Autodesk Inventor part; units mm, degrees
ref_plane "YZ Plane" through (0, 0, 0) normal (1, 0, 0) x (0, 1, 0)
ref_plane "XZ Plane" through (0, 0, 0) normal (0, 1, 0) x (-1, 0, 0)
ref_plane "XY Plane" through (0, 0, 0) normal (0, 0, 1) x (1, 0, 0)
sketch "Esquisse1" plane through (0, 0, 0) normal (0, 1, 0) x (-1, 0, 0)
  line L0 (-350, -500) -> (350, -500)
  line L1 (350, -500) -> (350, 500)
  line L2 (350, 500) -> (-350, 500)
  line L3 (-350, 500) -> (-350, -500)
  line L4 (-350, -500) -> (350, 500) construction
  line L5 (350, -500) -> (-350, 500) construction
  point P0 (0, 0)
  dimension "d0" = 1000
  dimension "d1" = 700
extrude "Extrusion1" add sketch "Esquisse1" along normal blind 18.55
sketch "Esquisse2" plane through (0, 18.55, 0) normal (0, 1, 0) x (1, 0, 0)
  line L0 (-350, 500) -> (-350, -500)
  line L1 (-350, -450) -> (-331.45, -450)
  line L2 (-331.45, -450) -> (-331.45, -350)
  line L3 (-331.45, -350) -> (-350, -350)
  line L4 (-350, -350) -> (-350, -450)
  line L5 (-350, -250) -> (-331.45, -250)
  line L6 (-331.45, -250) -> (-331.45, -150)
  line L7 (-331.45, -150) -> (-350, -150)
  line L8 (-350, -150) -> (-350, -250)
  line L9 (-350, -50) -> (-331.45, -50)
  line L10 (-331.45, -50) -> (-331.45, 50)
  line L11 (-331.45, 50) -> (-350, 50)
  line L12 (-350, 50) -> (-350, -50)
  line L13 (-350, 150) -> (-331.45, 150)
  line L14 (-331.45, 150) -> (-331.45, 250)
  line L15 (-331.45, 250) -> (-350, 250)
  line L16 (-350, 250) -> (-350, 150)
  line L17 (350, 500) -> (-350, 500)
  line L18 (-350, -500) -> (350, -500)
  line L19 (0, -500) -> (0, 500) construction
  line L20 (-350, 350) -> (-331.45, 350)
  line L21 (-331.45, 350) -> (-331.45, 450)
  line L22 (-331.45, 450) -> (-350, 450)
  line L23 (-350, 450) -> (-350, 350)
  line L24 (350, -450) -> (331.45, -450)
  line L25 (331.45, -450) -> (331.45, -350)
  line L26 (331.45, -350) -> (350, -350)
  line L27 (350, -350) -> (350, -450)
  line L28 (350, -250) -> (331.45, -250)
  line L29 (331.45, -250) -> (331.45, -150)
  line L30 (331.45, -150) -> (350, -150)
  line L31 (350, -150) -> (350, -250)
  line L32 (350, -50) -> (331.45, -50)
  line L33 (331.45, -50) -> (331.45, 50)
  line L34 (331.45, 50) -> (350, 50)
  line L35 (350, 50) -> (350, -50)
  line L36 (350, 150) -> (331.45, 150)
  line L37 (331.45, 150) -> (331.45, 250)
  line L38 (331.45, 250) -> (350, 250)
  line L39 (350, 250) -> (350, 150)
  line L40 (350, 350) -> (331.45, 350)
  line L41 (331.45, 350) -> (331.45, 450)
  line L42 (331.45, 450) -> (350, 450)
  line L43 (350, 450) -> (350, 350)
  point P0 (0, 0)
  point P1 (-350, -150)
  point P2 (-350, -250)
  point P3 (-350, 250)
  point P4 (-350, 150)
  point P5 (-350, -350)
  dimension "d6" = 18.55
  dimension "d9" = 200
  dimension "d26" = 50
  dimension "d27" = 100
  dimension "d32" = 50
extrude "Extrusion2" cut sketch "Esquisse2" against normal blind 18.55
properties part number "Plate"
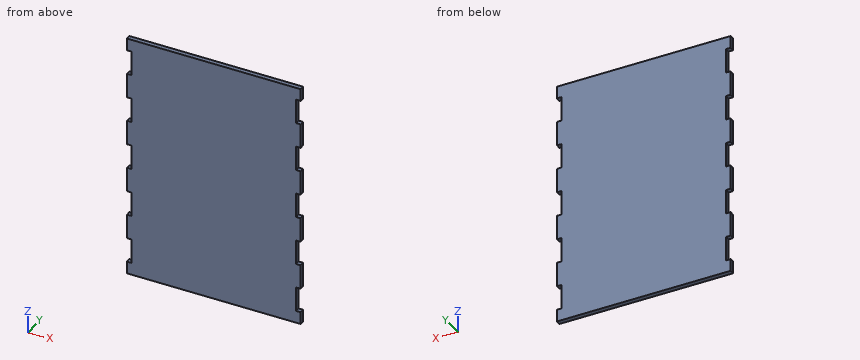
Could you check a few things on this model? Use its own coordinates, in mm. Round coordinates to 2 decimals unless told otherwise and drop trailing zeros. Loops run counter-clockwise (first coordinate to the right, second up) from the corner with the lowest first, then second, coordinate; pieces in that order, holes last.
Q1. I want a section at A-A (z = -224.5). Write out the boundary of the cut face in (x, y), and give its area (3 significant figures).
Q2. Please list where this line runs through material, in increasing order: L1, parallel to X at y = 9, z = 351.5.
Q3. For P1, Ø5.5, axis at y = 12, z = -210, coming from the -X side; P2, Ø9.5, axis at y = 10, z = 398.5, coming from the +X side, each with a flat end and sliding along its axis, tell me the tip position at first contact or that it passes through.
Answer below:
1. outline: (-331.45, 0) - (331.45, 0) - (331.45, 18.55) - (-331.45, 18.55) - close
1. area: 12,300 mm2
2. L1: x = -331.45 to 331.45
3. P1: stops at x = -331.45
3. P2: stops at x = 331.45
